from build123d import *

# Parameters (mm, degrees)
BOSS_EXTRUDE1_DEPTH = 2


with BuildPart() as part:
    # Sketch1 → Boss-Extrude1 (new body)
    with BuildSketch(Plane(origin=(0, 0, 0), x_dir=(-1, 0, 0), z_dir=(0, 0, -1))):
        with BuildLine():
            Line((-26.412606162, -93.321181126), (0.613755662, -63.832611026))
            Line((0.613755662, -63.832611026), (0.613755662, 50))
            Line((0.613755662, 50), (-504.386244338, 50))
            Line((-504.386244338, 50), (-504.386244338, -63.832611026))
            Line((-504.386244338, -63.832611026), (-477.359882514, -93.321181126))
            ThreePointArc((-477.359882514, -93.321181126), (-393.934701104, -89.753038855), (-336.886244338, -150.72816586))
            Line((-336.886244338, -150.72816586), (-166.886244338, -150.72816586))
            ThreePointArc((-166.886244338, -150.72816586), (-109.837787572, -89.753038855), (-26.412606162, -93.321181126))
        make_face()
    extrude(amount=-BOSS_EXTRUDE1_DEPTH)


solid = part.part
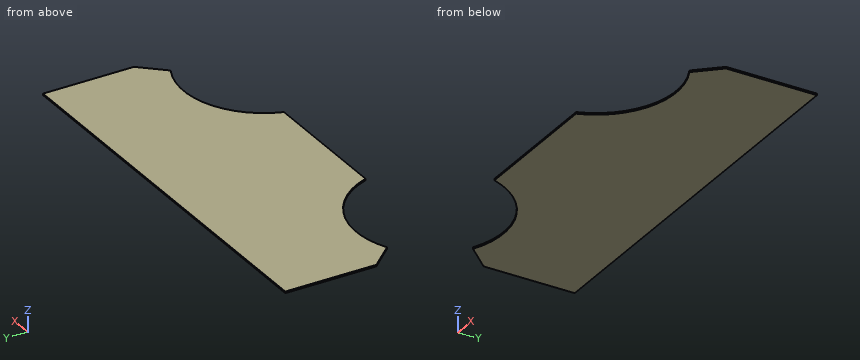
The model under review builds one solid part; all positions refer to its coordinate system, in mm. Give positions to 0.01 mm unless a question says otherwise; leave off trailing zeros. Order: outer loops, then holes, each group sorted by start corner. A loop starts at its lowest first (then second) coordinate and runs counter-clockwise, first axis right, second up. Notation, with made-up numbers: M 63,-36 L 85,-36 A12 cw 85,-14 Z; hole C -13.75,72.5 d7. An arc over 180 degrees is marked long. Use one line per item in the form item = value. Start each with the question number.
Item 1: We need section B-B on x = 438. Give the boundary of the cut face in (y, z).
Item 2: We need section C-C on y = -105.5. Give the boundary of the cut face in (x, z).
Item 3: We need section A-A on z = 1.25. Give the boundary of the cut face in (x, y), plus the area to 3 significant figures.
Item 4: To check wall thickness, follow line 1 along Y through (x, z) = (409.5, 0.9); line 2 along Y through (x, z) = (445, 0.1); line 3 along X through (y, z) = (-134, 0.2). State the ranges of each line that lie inside material, in increasing order. Write a range as from..to.
Completed:
q1.outline = M -82.52,0 L 50,0 L 50,2 L -82.52,2 Z
q2.outline = M 136.03,0 L 367.75,0 L 367.75,2 L 136.03,2 Z
q3.outline = M -0.61,-63.83 L 26.41,-93.32 A100 cw 166.89,-150.73 L 336.89,-150.73 A100 cw 477.36,-93.32 L 504.39,-63.83 L 504.39,50 L -0.61,50 Z
q3.area = 82,100 mm²
q4.line_1 = -84.83..50
q4.line_2 = -83.2..50
q4.line_3 = 159.56..344.21
